from build123d import *

# Parameters (mm, degrees)
SKETCH1_W           = 63.5
SKETCH1_H           = 245.9736
SKETCH1_R           = 7.9375
BOSS_EXTRUDE1_DEPTH = 3.048
CHAMFER1_SIZE       = 2.54


with BuildPart() as part:
    # Sketch1 → Boss-Extrude1 (new body)
    with BuildSketch(Plane.XY):
        with Locations((31.75, 122.9868)):
            Rectangle(SKETCH1_W, SKETCH1_H)
        with Locations((31.75, 192.3796)):
            Circle(SKETCH1_R, mode=Mode.SUBTRACT)
    extrude(amount=BOSS_EXTRUDE1_DEPTH)

    # Chamfer1
    chamfer1_edges = [part.edges().sort_by_distance(p)[0] for p in [
        (0, 245.9736, 1.524),
        (63.5, 245.9736, 1.524),
    ]]
    chamfer(chamfer1_edges, length=CHAMFER1_SIZE)


solid = part.part
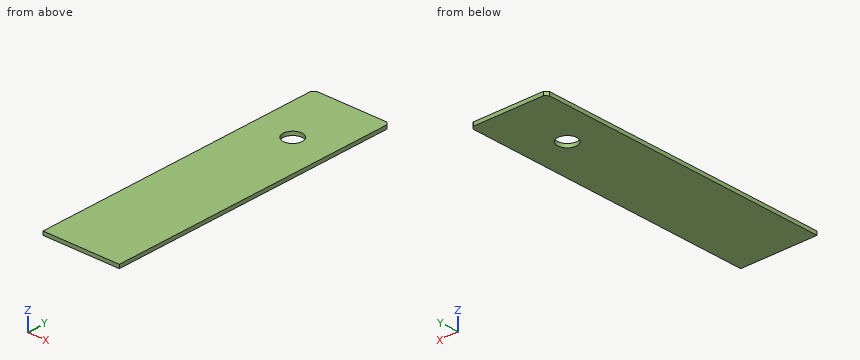
The listing builds one solid part. Answer for the finished solid, in the listing's coordinates (mm). Give positions to 0.01 mm unless a question says otherwise; leave off trailing zeros. Order: outer loops, then holes, each group sorted by start corner. A loop starts at its lowest first (then second) coordinate and runs counter-clockwise, first axis right, second up. Notation, with made-up numbers: (78.5, 8) - (102.5, 8) arc R15 ccw to (102.5, 35) - close; hole circle Ø5 at (-38, -27). An arc over 180 degrees is marked (long way). Use one line per item in the form item = value.
1) Consider probe 1 along Y at (x, z) = (31.75, 1.6); probe 2 along Y at (x, z) = (29.5, 0.5). Determine where each line is inside the solid, lowest interval first. Write a range as [from, to].
Verdict:
probe_1 = [0, 184.44], [200.32, 245.97]
probe_2 = [0, 184.77], [199.99, 245.97]
2) Find section A-A on x = 31.75. Determine the outline of the cut face in (y, z), and give its area (3 significant figures).
Verdict:
outline = (0, 0) - (184.44, 0) - (184.44, 3.05) - (0, 3.05) - close; (200.32, 0) - (245.97, 0) - (245.97, 3.05) - (200.32, 3.05) - close
area = 701 mm^2
3) Each of these flat-tipped pins is pushed along its axis until it touches: pin 1 (12.5 mm diameter, centred on x = 31.75, y = 192.38, fed in from -Z); pin 2 (1.5 mm diameter, centred on x = 52.5, y = 98.5, fed in from -Z). Where does it stop, or does it pass through?
Verdict:
pin_1 = through
pin_2 = 0
